```python
from build123d import *

# Parameters (mm, degrees)
ESQUISSE2_R                  = 1.25
ENL_V_MAT_EXTRU_1_DEPTH      = 33.372828112
TROU_TARAUD_M41_D            = 3.3
R_P_TITION_CIRCULAIRE1_COUNT = 3
CHANFREIN1_SIZE              = 0.6


with BuildPart() as part:
    # Esquisse1 → Révolution1 (revolve)
    with BuildSketch(Plane.XY, mode=Mode.PRIVATE) as r_volution1_sk:
        Polygon((0, 2), (20, 2), (20, 18), (15, 18), (15, 7.5), (9, 7.5), (9, 4), (0, 4), align=None)
    revolve(r_volution1_sk.sketch.rotate(Axis((0, 0, 0), (1, 0, 0)), 90), axis=Axis((0, 0, 0), (1, 0, 0)))

    # Esquisse2 → Enlèv. mat.-Extru.1 (cut, through all)
    with BuildSketch(Plane.XY):
        with Locations((12, 0)):
            Circle(ESQUISSE2_R)
    extrude(amount=-ENL_V_MAT_EXTRU_1_DEPTH, mode=Mode.SUBTRACT)

    # Trou taraudé M41 (through all)
    with Locations(Plane(origin=(20, 0, 0), x_dir=(0, 0, -1), z_dir=(1, 0, 0))):
        with Locations((0, 12)):
            trou_taraud_m41 = Hole(TROU_TARAUD_M41_D / 2)

    # Répétition circulaire1: Trou taraudé M41 ×3 about axis
    r_p_tition_circulaire1_axis = Axis((0, 0, 0), (1, 0, 0))
    for i in range(1, R_P_TITION_CIRCULAIRE1_COUNT):
        add(trou_taraud_m41.rotate(r_p_tition_circulaire1_axis, i * 360 / R_P_TITION_CIRCULAIRE1_COUNT), mode=Mode.SUBTRACT)

    # Chanfrein1
    chanfrein1_edges = [part.edges().sort_by_distance(p)[0] for p in [
        (20, 0, -18),
    ]]
    chamfer(chanfrein1_edges, length=CHANFREIN1_SIZE)


solid = part.part
```
Geometry check sheet. Reference: the model listing, model coordinates, mm. A direction names the side the tool comes from. Round coordinates to 2 decimals unless told otherwise and drop trailing zeros. Loops run counter-clockwise (first coordinate to the right, second up) from the corner with the lowest first, then second, coordinate; pieces in that order, holes last. Notation, with made-up numbers: M -2,68.25 L 22,68.25 A6 ccw 22,78.25 Z; hole C 38.5,50.5 d6. An arc over 180 degrees is marked long. Return JSON: item names as keys, results as strings. Group by question number.
(1) Section check A-A, the plane z = 0. Enter the section's corners in (x, y), and give its area (3 significant figures).
(2) Mould release check, pull along X, two halves, no side actions. Record for faces 1 (the face through (17.465, -7.004, -11.702)), 2 (the face through (11.84, 1.24, -4.49)), 3 (the face through (0, 1, -2)): pulls with the +X half, pulls with the -X half, needs draft (parallel to the pull), parting line crosses it, or undercut.
(3) Section check C-C, the plane x = 14.5. Enter the section's corners in (y, z), and give its area (3 significant figures).
(4) Go/stop test with flat-tipped pins: pin 1 (1.5 mm diameter, centred on x = 13, z = 13, fed in from -Y); pin 2 (3 mm diameter, centred on x = 12, y = 0, fed in from +Z); pin 3 (5.5 mm diameter, centred on y = -6, z = 10.39, fed in from -X); pin 4 (10 mm diameter, centred on x = 8, y = 11, fed in from -Z). Record where each tip stops, or that it passes through.
(5) Section check D-D, the plane x = 5.5. Enter the section's corners in (y, z), and give its area (3 significant figures).
(6) Section check B-B, the plane y = 0. Enter the section's corners in (x, z), and give its area (3 significant figures).
(7) Set-up check for faces 4 (the face through (17.169, -12.165, -13.267)), 5 (the face through (9, 3, 3)): record each of +Z, -Z, +X, -X, +Y, -Y from which the full face is reachable in a straight line by a thin tool's end or side.
(8) Scan lines: line 1 along Y through (x, z) = (15.5, 0); line 2 along X through (y, z) = (8, 8.5); line 3 along Y through (x, z) = (18.75, -1). Record each from-to range of solid material in increasing order. Write a range as [from, to].
Data:
{
 "1": {"outline": "M 0,-4 L 9,-4 L 9,-7.5 L 15,-7.5 L 15,-18 L 19.4,-18 L 20,-17.4 L 20,-2 L 0,-2 Z; M 0,2 L 20,2 L 20,10.35 L 15,10.35 L 15,7.5 L 9,7.5 L 9,4 L 0,4 Z; M 15,13.65 L 20,13.65 L 20,17.4 L 19.4,18 L 15,18 Z", "area": "245 mm²"},
 "2": {"face 1": "needs draft", "face 2": "undercut", "face 3": "pulls with the -X half"},
 "3": {"outline": "C 0,0 d15; hole C 0,0 d4", "area": "164 mm²"},
 "4": {"pin 1": "through", "pin 2": "z = 7.5", "pin 3": "x = 15", "pin 4": "z = -4.36"},
 "5": {"outline": "C 0,0 d8; hole C 0,0 d4", "area": "37.7 mm²"},
 "6": {"outline": "M 0,-4 L 9,-4 L 9,-7.5 L 10.75,-7.5 L 10.75,-2 L 0,-2 Z; M 0,2 L 20,2 L 20,17.4 L 19.4,18 L 15,18 L 15,7.5 L 9,7.5 L 9,4 L 0,4 Z; M 13.25,-7.5 L 15,-7.5 L 15,-18 L 19.4,-18 L 20,-17.4 L 20,-2 L 13.25,-2 Z", "area": "248 mm²"},
 "7": {"face 4": "+X, -X", "face 5": "-X"},
 "8": {"line 1": "[-18, -2], [2, 10.35], [13.65, 18]", "line 2": "[15, 20]", "line 3": "[-17.97, -1.73], [1.73, 10.69], [13.31, 17.97]"}
}
